Verification items for the finished model (mm, model axes). Face numbers are marked on the shaded views. A direction names the side the tool comes from. Coordinates: 2 decimals unless noted, no trailing zeros. Order: outer loops, then holes, each group sorted by start corner. A loop starts at its lowest first (then second) coordinate and runs counter-clockwise, first axis right, second up.
Q1. Thickness scan on line 1 (Y direction, x = -50, z = -5.5); line 2 (X direction, y = 3, z = -11); line 3 (X direction, y = 11, z = 24). Record the ranges inside material, lowest first.
Q2. Set-up check for the marked faces 1 and 2: record each of +Z, -Z, +X, -X, +Y, -Y from which the full face is reachable in a straight line by a thin tool's end or side.
Q3. Cross-section at B-B, the plane x = 31.75. Record the boundary of the cut face in (y, z).
Q4. Cross-section at D-D, the plane x = -10. Record the boundary of the cut face in (y, z), and give its area (3 significant figures).
Q5. Depth check by flat-ended pin: P1, Ø2.5, axis at x = -14, y = 1, coming from the +Z side; P2, Ø2, axis at x = 22.5, z = 22.5, coming from the +Y side; P3, Ø3.5, axis at x = -38, y = 1.5, coming from the -Z side; P4, Ø5, axis at x = -8, y = 8, coming from the +Z side. Enter the tip coordinate at first touch or a pass-through.
Q6. Cross-section at A-A, the plane x = -39.5. Record the boundary of the cut face in (y, z).
Q7. Cross-section at C-C, the plane z = 25.5. Record the boundary of the cut face in (x, y).
from build123d import *

# Parameters (mm, degrees)
EXTRUDE_1_DEPTH     = 4.6
SKETCH_1_R          = 2.625
SKETCH_1_W          = 40.4
SKETCH_1_H          = 4.6
CUT_EXTRUDE_1_DEPTH = 4.6
SKETCH_5_R          = 7.5
EXTRUDE_2_DEPTH     = 7
SKETCH_6_R          = 2.6
EXTRUDE_3_DEPTH     = 8
FILLET_1_R          = 5
FILLET_2_R          = 4


with BuildPart() as part:
    # 草图3 → 凸台-拉伸1 (new body)
    with BuildSketch(Plane(origin=(0, 0, 0), x_dir=(1, 0, 0), z_dir=(0, 1, 0))):
        Polygon((-40, 28), (-60, 28), (-60, -28), (-40, -28), (18.5, -28), (18.5, -36), (45, -36), (45, -28), (45, 28), (45, 36), (18.5, 36), (18.5, 28), align=None)
    extrude(amount=EXTRUDE_1_DEPTH)

    # 草图1 → 切除-拉伸1 (cut)
    with BuildSketch(Plane(origin=(0, 0, 0), x_dir=(1, 0, 0), z_dir=(0, 1, 0))):
        with Locations(Location((-31.75, 20.6375, 0), (0, 0, 270))):
            Circle(SKETCH_1_R)
        with Locations(Location((31.75, 20.6375, 0), (0, 0, 90))):
            Circle(SKETCH_1_R)
        with Locations(Location((31.75, -20.6375, 0), (0, 0, 270))):
            Circle(SKETCH_1_R)
        with Locations(Location((-31.75, -20.6375, 0), (0, 0, 90))):
            Circle(SKETCH_1_R)
        with Locations((-28, -10.4375)):
            Rectangle(SKETCH_1_W, SKETCH_1_H)
        with Locations((-28, 10.4375)):
            Rectangle(SKETCH_1_W, SKETCH_1_H)
        Polygon((-22.25, -26.5375), (-22.25, -14.7375), (-0.65, -14.7375), (-0.65, -26.5375), (-0.65, -30.009482824), (-22.25, -30.009482824), align=None)
        Polygon((-22.25, 14.7375), (-0.65, 14.7375), (-0.65, 26.5375), (-0.65, 30.009482824), (-22.25, 30.009482824), (-22.25, 26.5375), align=None)
    extrude(amount=CUT_EXTRUDE_1_DEPTH, mode=Mode.SUBTRACT)

    # 草图5 → 凸台-拉伸2 (add)
    with BuildSketch(Plane(origin=(0, 4.6, 0), x_dir=(1, 0, 0), z_dir=(0, 1, 0))):
        with Locations(Location((31.75, -20.6375, 0), (0, 0, 270))):
            Circle(SKETCH_5_R)
    extrude(amount=EXTRUDE_2_DEPTH)

    # 草图6 → 凸台-拉伸3 (add)
    with BuildSketch(Plane(origin=(0, 11.6, 0), x_dir=(1, 0, 0), z_dir=(0, 1, 0))):
        with Locations(Location((31.75, -20.6375, 0), (0, 0, 270))):
            Circle(SKETCH_6_R)
    extrude(amount=EXTRUDE_3_DEPTH)

    # 圆角1
    fillet_1_edges = [part.edges().sort_by_distance(p)[0] for p in [
        (-22.25, 2.3, 14.7375),
        (-0.65, 2.3, 14.7375),
        (-0.65, 2.3, -14.7375),
        (-22.25, 2.3, -14.7375),
    ]]
    fillet(fillet_1_edges, radius=FILLET_1_R)

    # 圆角2
    fillet_2_edges = [part.edges().sort_by_distance(p)[0] for p in [
        (-0.65, 2.3, 28),
        (-22.25, 2.3, 28),
        (-0.65, 2.3, -28),
        (-22.25, 2.3, -28),
        (-60, 2.3, 28),
        (-60, 2.3, -28),
        (18.5, 2.3, -28),
        (18.5, 2.3, -36),
        (45, 2.3, -36),
        (45, 2.3, 36),
        (18.5, 2.3, 36),
        (18.5, 2.3, 28),
    ]]
    fillet(fillet_2_edges, radius=FILLET_2_R - 0.0001)  # a hair under: the kernel refuses the full size


solid = part.part
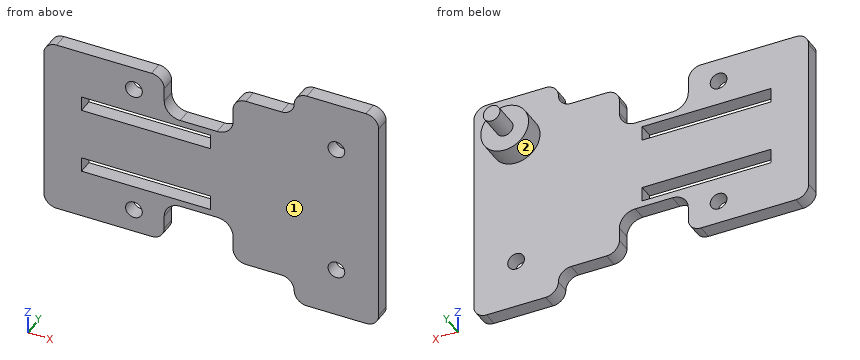
Check values:
1. line 1: y = 0 to 4.6
1. line 2: x = -60 to -48.2, -7.8 to 45
1. line 3: x = 25.05 to 38.45
2. face 1: +Z, -Z, +X, -X, -Y
2. face 2: +Y
3. outline: (0, -36) - (4.6, -36) - (4.6, -23.26) - (0, -23.26) - close; (0, -18.01) - (4.6, -18.01) - (4.6, 13.14) - (11.6, 13.14) - (11.6, 18.04) - (19.6, 18.04) - (19.6, 23.24) - (11.6, 23.24) - (11.6, 28.14) - (4.6, 28.14) - (4.6, 36) - (0, 36) - (0, 23.26) - (4.6, 23.26) - (4.6, 18.01) - (0, 18.01) - close
4. outline: (0, -14.74) - (4.6, -14.74) - (4.6, -12.74) - (0, -12.74) - close; (0, -8.14) - (4.6, -8.14) - (4.6, 8.14) - (0, 8.14) - close; (0, 12.74) - (4.6, 12.74) - (4.6, 14.74) - (0, 14.74) - close
4. area: 93.3 mm2
5. P1: stops at z = 14.74
5. P2: stops at y = 4.6
5. P3: stops at z = -28
5. P4: passes through
6. outline: (0, -28) - (4.6, -28) - (4.6, -12.74) - (0, -12.74) - close; (0, -8.14) - (4.6, -8.14) - (4.6, 8.14) - (0, 8.14) - close; (0, 12.74) - (4.6, 12.74) - (4.6, 28) - (0, 28) - close
7. outline: (-59.71, 0) - (-22.54, 0) - (-22.54, 4.6) - (-59.71, 4.6) - close; (-0.36, 0) - (45, 0) - (45, 4.6) - (37.46, 4.6) - (37.46, 11.6) - (26.04, 11.6) - (26.04, 4.6) - (-0.36, 4.6) - close
